```python
from build123d import *

# Parameters (mm, degrees)
F0_W     = 120
F0_H     = 115
F1_DEPTH = 15
F2_W     = 100
F2_H     = 15
F3_DEPTH = 15.001
F4_R     = 2.5
F5_DEPTH = 120.001
F6_SIZE2 = 14.99999
F6_SIZE  = 89.99999
F7_R     = 7.49999


# Not quite as in the source:
# - a fillet or chamfer is up to 0.001 mm smaller than in the source, because OpenCascade refuses the exact size


with BuildPart() as f1:
    # F0 (on Top) → F1 (new body)
    with BuildSketch(Plane.XY):
        Rectangle(F0_W, F0_H)
    extrude(amount=F1_DEPTH)

    # F2 (on face) → F3 (cut, through all)
    with BuildSketch(Plane.XY.offset(15)):
        with Locations((0, 50)):
            Rectangle(F2_W, F2_H)
    extrude(amount=-F3_DEPTH, mode=Mode.SUBTRACT)

    # F4 (on face) → F5 (cut, through all)
    with BuildSketch(Plane.YZ.offset(60)):
        with Locations((50, 7.5)):
            Circle(F4_R)
    extrude(amount=-F5_DEPTH, mode=Mode.SUBTRACT)

    # F6 (size 90 and 15 in the source; OpenCascade refuses exactly that, so slightly less here)
    f6_edges = [f1.edges().sort_by_distance(p)[0] for p in [
        (0, -57.5, 15),
    ]]
    f6_side = f1.faces().sort_by_distance((0, -6.097561, 15))[0]
    chamfer(f6_edges, length=F6_SIZE, length2=F6_SIZE2, reference=f6_side)

    # F7 (radius 7.5 in the source; OpenCascade refuses exactly that, so slightly less here)
    f7_edges = [f1.edges().sort_by_distance(p)[0] for p in [
        (55, 57.5, 15),
        (55, 57.5, 0),
        (-55, 57.5, 0),
        (-55, 57.5, 15),
    ]]
    fillet(f7_edges, radius=F7_R)


solid = f1.part
```
The model under review builds one solid part; all positions refer to its coordinate system, in mm. A direction names the side the tool comes from. Round coordinates to 2 decimals unless told otherwise and drop trailing zeros. Order: outer loops, then holes, each group sorted by start corner. A loop starts at its lowest first (then second) coordinate and runs counter-clockwise, first axis right, second up.
Item 1: Add section C-C, the plane z = 11.5. State the section outline as (x, y) points.
Working result:
outline: (-60, 11.5) - (60, 11.5) - (60, 56.34) - (50, 56.34) - (50, 42.5) - (-50, 42.5) - (-50, 56.34) - (-60, 56.34) - close
Item 2: For pin 1 (4.5 mm diameter, centred on x = 24.5, z = 6, fed in from +Y), flat-tipped, find the tip position at first contact; note if it passes through.
Working result:
pin 1: stops at y = 42.5
Item 3: Machinability: for faces 1 (the flat face through (50, 47, 8)), 2 (the flat face through (-0.8, -13.1, 7.4)), which of the approach directions +Z, -Z, +X, -X, +Y, -Y give a long, thin tool a straight path to every point of the face, cutting with its end or side? Answer none if there is none.
Working result:
face 1: +Z, -Z, +Y
face 2: +Z, +X, -X, -Y
Item 4: To check wall thickness, follow probe 1 along Z at (x, y) = (52.5, 50); probe 2 along X at (y, z) = (50, 12.75); probe 3 along Z at (x, y) = (4, -34). State the ranges of each line that lie inside material, in increasing order.
Working result:
probe 1: z = 0 to 5, 10 to 15
probe 2: x = -60 to -50, 50 to 60
probe 3: z = 0 to 3.92
Item 5: Draft analysis for pull direction Y (two halves, no side actions). For faces 3 (the cylindrical face through (55.07, 52.31, 6.54)), 4 (the cylindrical face through (-54.93, 55.245, 2.139)), 5 (the flat face through (-50, 47, 8)), state which applies: released by +Y, released by -Y, zero draft, split by the parting line, or undercut.
Working result:
face 3: undercut
face 4: released by +Y
face 5: zero draft
Item 6: Add section B-B, the plane y = 44.5. State the section outline as (x, z) points, and give its area (3 significant figures).
Working result:
outline: (-60, 0) - (-50, 0) - (-50, 15) - (-60, 15) - close; (50, 0) - (60, 0) - (60, 15) - (50, 15) - close
area: 300 mm2
